from build123d import *

# Parameters (mm, degrees)
SKETCH1_R          = 1.7
CUT_EXTRUDE1_DEPTH = 69.450712195
CIRPATTERN1_COUNT  = 4


with BuildPart() as part:
    # Croquis2 → Revolución1 (revolve)
    with BuildSketch(Plane(origin=(0, 0, 0), x_dir=(1, 0, 0), z_dir=(0, 1, 0)), mode=Mode.PRIVATE) as revoluci_n1_sk:
        Polygon((25, -19), (25, 0), (35, 0), (35, -7), (46.5, -7), (46.5, -19), align=None)
    revolve(revoluci_n1_sk.sketch.rotate(Axis((0, 0, -25.844178122), (0, 0, 1)), 180), axis=Axis((0, 0, -25.844178122), (0, 0, 1)))

    # Sketch1 → Cut-Extrude1 (cut, symmetric)
    with BuildSketch(Plane.XY.offset(19)):
        with Locations((0, 30)):
            Circle(SKETCH1_R)
    cut_extrude1 = extrude(amount=CUT_EXTRUDE1_DEPTH, both=True, mode=Mode.SUBTRACT)

    # CirPattern1: Cut-Extrude1 ×4 about axis
    cirpattern1_axis = Axis((0, 0, 0), (0, 0, 1))
    for i in range(1, CIRPATTERN1_COUNT):
        add(cut_extrude1.rotate(cirpattern1_axis, i * 360 / CIRPATTERN1_COUNT), mode=Mode.SUBTRACT)


solid = part.part
Could you check a few things on this model? Use its own coordinates, in mm. A direction names the side the tool comes from. Give positions to 0.01 mm unless a question says otherwise; leave off trailing zeros. Order: outer loops, then holes, each group sorted by start corner. A loop starts at its lowest first (then second) coordinate and runs counter-clockwise, first axis right, second up.
1. Suppose I cut it at D-D (x = 30). Write out the boundary of the cut face in (y, z).
Answers below:
outline: (-35.53, 7) - (-18.03, 7) - (-18.03, 0) - (-1.7, 0) - (-1.7, 19) - (-35.53, 19) - close; (1.7, 0) - (18.03, 0) - (18.03, 7) - (35.53, 7) - (35.53, 19) - (1.7, 19) - close
2. Which directions (+Z, -Z, +X, -X, +Y, -Y) give clear straight access to the entire face, cutting with the end or side of a thin tool? Please do faces 1 (the flat face through (7, -35, 7)), 2 (the cylindrical face through (-28.34, -0.37, 9.63)).
Answers below:
face 1: -Z
face 2: +Z, -Z
3. I need wall thicknesses on L1, parallel to Y at x = 0, z = 13.75; L2, parallel to X at y = 19, z = 14.5; L3, parallel to Y at x = 16.5, z = 18.25. Which ranges of each line are inside material? Lowest first, please.
Answers below:
L1: y = -46.5 to -31.7, -28.3 to -25, 25 to 28.3, 31.7 to 46.5
L2: x = -42.44 to -16.25, 16.25 to 42.44
L3: y = -43.47 to -18.78, 18.78 to 43.47
4. Suppose I cut it at B-B (z = 12). Write out the boundary of the cut face in (x, y), plus the area to 3 significant figures.
Answers below:
outline: circle Ø93 at (0, 0); hole circle Ø3.4 at (-30, 0); hole circle Ø50 at (0, 0); hole circle Ø3.4 at (0, -30); hole circle Ø3.4 at (0, 30); hole circle Ø3.4 at (30, 0)
area: 4,790 mm2
5. Suppose I cut it at A-A (x = 0). Write out the boundary of the cut face in (y, z).
Answers below:
outline: (-46.5, 7) - (-35, 7) - (-35, 0) - (-31.7, 0) - (-31.7, 19) - (-46.5, 19) - close; (-28.3, 0) - (-25, 0) - (-25, 19) - (-28.3, 19) - close; (25, 0) - (28.3, 0) - (28.3, 19) - (25, 19) - close; (31.7, 0) - (35, 0) - (35, 7) - (46.5, 7) - (46.5, 19) - (31.7, 19) - close
6. Suppose I cut it at C-C (y = -11). Write out the boundary of the cut face in (x, z), plus the area to 3 significant figures.
Answers below:
outline: (-45.18, 7) - (-33.23, 7) - (-33.23, 0) - (-22.45, 0) - (-22.45, 19) - (-45.18, 19) - close; (22.45, 0) - (33.23, 0) - (33.23, 7) - (45.18, 7) - (45.18, 19) - (22.45, 19) - close
area: 696 mm2
7. Thinking about a two-plate mould opening in X: for faces 3 (the cylindrical face through (7.587, 34.168, 3.549)), 4 (the flat face through (23, -11, 0)), 5 (the cylindrical face through (28.34, 0.37, 9.63)), which applies, +X half, -X half, draft (parallel to the pull), parting line (faces both ways), or undercut?
Answers below:
face 3: parting line
face 4: draft
face 5: undercut
8. For pin 1 (2 mm diameter, centred on x = 20.5, y = 10, fed in from +Z); pin 2 (10 mm diameter, centred on y = 8, z = 9, fed in from +X); pin 3 (10 mm diameter, centred on y = 30, z = 8.5, fed in from -X); pin 4 (8 mm diameter, centred on x = 31, z = 15.5, fed in from -Y), each with a flat end and sliding along its axis, tell me the tip position at first contact or that it passes through.
Answers below:
pin 1: passes through
pin 2: stops at x = 46.4
pin 3: stops at x = -39.21
pin 4: stops at y = -37.86
